from build123d import *

# Parameters (mm, degrees)
F1_DEPTH = 5.08
F2_SIZE  = 5.07999


# Not quite as in the source:
# - a fillet or chamfer is up to 0.001 mm smaller than in the source, because OpenCascade refuses the exact size


with BuildPart() as f1:
    # F0 (on Top) → F1 (new body)
    with BuildSketch(Plane.XY):
        with BuildLine():
            ThreePointArc((-6.4398498965, 10.9461560975), (-3.3372007403, 12.2536970429), (0, 12.7))
            Line((0, 12.7), (0, 38.1))
            Line((0, 38.1), (-11.0489271221, 18.7804503105))
            Line((-11.0489271221, 18.7804503105), (-6.4398498965, 10.9461560975))
        make_face()
        with BuildLine():
            ThreePointArc((0, 12.7), (3.261881723, 12.2739613665), (6.304915, 11.0244295473))
            Line((6.304915, 11.0244295473), (10.9721234563, 19.185255))
            Line((10.9721234563, 19.185255), (0, 38.1))
            Line((0, 38.1), (0, 12.7))
        make_face()
        with BuildLine():
            ThreePointArc((-2.7338674235, 4.6469001683), (-1.4167200379, 5.2019819875), (0, 5.3914480674))
            Line((0, 5.3914480674), (0, 12.7))
            ThreePointArc((0, 12.7), (-3.3372007403, 12.2536970429), (-6.4398498965, 10.9461560975))
            Line((-6.4398498965, 10.9461560975), (-2.7338674235, 4.6469001683))
        make_face()
        with BuildLine():
            ThreePointArc((0, 5.3914480674), (1.3847453474, 5.2105846684), (2.6765843931, 4.6801290848))
            Line((2.6765843931, 4.6801290848), (6.304915, 11.0244295473))
            ThreePointArc((6.304915, 11.0244295473), (3.261881723, 12.2739613665), (0, 12.7))
            Line((0, 12.7), (0, 5.3914480674))
        make_face()
        with BuildLine():
            ThreePointArc((-5.3914480674, 0), (-4.6801290848, 2.6765843931), (-2.7338674235, 4.6469001683))
            Line((-2.7338674235, 4.6469001683), (-6.4398498965, 10.9461560975))
            ThreePointArc((-6.4398498965, 10.9461560975), (-11.0244295473, 6.304915), (-12.7, 0))
            Line((-12.7, 0), (-5.3914480674, 0))
        make_face()
        with BuildLine():
            ThreePointArc((2.6765843931, 4.6801290848), (4.6636025783, 2.7052769276), (5.3914480674, 0))
            Line((5.3914480674, 0), (12.7, 0))
            ThreePointArc((12.7, 0), (10.9855, 6.3725026285), (6.304915, 11.0244295473))
            Line((6.304915, 11.0244295473), (2.6765843931, 4.6801290848))
        make_face()
        with BuildLine():
            Line((-10.9461560975, -6.4398498965), (-4.6469001683, -2.7338674235))
            ThreePointArc((-4.6469001683, -2.7338674235), (-5.2019819875, -1.4167200379), (-5.3914480674, 0))
            Line((-5.3914480674, 0), (-12.7, 0))
            ThreePointArc((-12.7, 0), (-12.2536970429, -3.3372007403), (-10.9461560975, -6.4398498965))
        make_face()
        with BuildLine():
            Line((12.7, 0), (5.3914480674, 0))
            ThreePointArc((5.3914480674, 0), (5.2105846684, -1.3847453474), (4.6801290848, -2.6765843931))
            Line((4.6801290848, -2.6765843931), (11.0244295473, -6.304915))
            ThreePointArc((11.0244295473, -6.304915), (12.2739613665, -3.261881723), (12.7, 0))
        make_face()
        with BuildLine():
            Line((11.0244295473, -6.304915), (4.6801290848, -2.6765843931))
            ThreePointArc((4.6801290848, -2.6765843931), (3.835671013, -3.7888441699), (2.7338674235, -4.6469001683))
            Line((2.7338674235, -4.6469001683), (6.4398498965, -10.9461560975))
            ThreePointArc((6.4398498965, -10.9461560975), (9.0352390037, -8.9249345178), (11.0244295473, -6.304915))
        make_face()
        with BuildLine():
            Line((6.4398498965, -10.9461560975), (2.7338674235, -4.6469001683))
            ThreePointArc((2.7338674235, -4.6469001683), (0.0331115783, -5.3913463891), (-2.6765843931, -4.6801290848))
            Line((-2.6765843931, -4.6801290848), (-6.304915, -11.0244295473))
            ThreePointArc((-6.304915, -11.0244295473), (0.07799705, -12.6997604883), (6.4398498965, -10.9461560975))
        make_face()
        with BuildLine():
            ThreePointArc((-2.6765843931, -4.6801290848), (-3.7888441699, -3.835671013), (-4.6469001683, -2.7338674235))
            Line((-4.6469001683, -2.7338674235), (-10.9461560975, -6.4398498965))
            ThreePointArc((-10.9461560975, -6.4398498965), (-8.9249345178, -9.0352390037), (-6.304915, -11.0244295473))
            Line((-6.304915, -11.0244295473), (-2.6765843931, -4.6801290848))
        make_face()
        with BuildLine():
            Line((-32.8384682925, -19.3195496895), (-10.9461560975, -6.4398498965))
            ThreePointArc((-10.9461560975, -6.4398498965), (-12.2536970429, -3.3372007403), (-12.7, 0))
            Line((-12.7, 0), (-21.7895411704, 0))
            Line((-21.7895411704, 0), (-32.8384682925, -19.3195496895))
        make_face()
        with BuildLine():
            ThreePointArc((-6.304915, -11.0244295473), (-8.9249345178, -9.0352390037), (-10.9461560975, -6.4398498965))
            Line((-10.9461560975, -6.4398498965), (-32.8384682925, -19.3195496895))
            Line((-32.8384682925, -19.3195496895), (-10.9721234563, -19.185255))
            Line((-10.9721234563, -19.185255), (-6.304915, -11.0244295473))
        make_face()
        with BuildLine():
            Line((33.0732886418, -18.914745), (11.0244295473, -6.304915))
            ThreePointArc((11.0244295473, -6.304915), (9.0352390037, -8.9249345178), (6.4398498965, -10.9461560975))
            Line((6.4398498965, -10.9461560975), (11.2069438057, -19.0490396895))
            Line((11.2069438057, -19.0490396895), (33.0732886418, -18.914745))
        make_face()
        with BuildLine():
            Line((22.1011651855, 0), (12.7, 0))
            ThreePointArc((12.7, 0), (12.2739613665, -3.261881723), (11.0244295473, -6.304915))
            Line((11.0244295473, -6.304915), (33.0732886418, -18.914745))
            Line((33.0732886418, -18.914745), (22.1011651855, 0))
        make_face()
    extrude(amount=F1_DEPTH)

    # F2 (size 5.08 in the source; OpenCascade refuses exactly that, so slightly less here)
    f2_edges = [f1.edges().sort_by_distance(p)[0] for p in [
        (-5.524464, 28.440225, 5.08),
        (5.486062, 28.642628, 5.08),
        (-27.314005, -9.659775, 5.08),
        (-21.905296, -19.252402, 5.08),
        (22.140116, -18.981892, 5.08),
        (27.587227, -9.457373, 5.08),
    ]]
    chamfer(f2_edges, length=F2_SIZE)


solid = f1.part
For this review, take the finished solid that the model builds, in its own axes (mm). A direction names the side the tool comes from. Coordinates: 2 decimals unless noted, no trailing zeros. Order: outer loops, then holes, each group sorted by start corner. A loop starts at its lowest first (then second) coordinate and runs counter-clockwise, first axis right, second up. Notation, with made-up numbers: (23, -31.5) - (38, -31.5) arc R24 ccw to (38, -13.5) - close; hole circle Ø7 at (49.25, 61). An arc over 180 degrees is marked (long way). Answer as CSV lines item,"result". Start each with the question number.
1) To check wall thickness, follow line 1 along X through (y, z) = (-4, 2.25); line 2 along X through (y, z) = (-4.5, 1.6); line 3 along Z through (x, y) = (24, -8.5). State the ranges of each line that lie inside material, in increasing order. Write a range as [from, to].
2) Machinability: for faces 1 (the flat face through (-8.153, -14.255, 1.94)), 2 (the cylindrical face through (-10.98, 6.38, 2.5)), 3 (the flat face through (8.087, 14.141, 1.94)), 4 (the flat face through (16, 0, 2)), which of the approach directions +Z, -Z, +X, -X, +Y, -Y give a long, thin tool a straight path to every point of the face, cutting with its end or side? Answer none if there is none.
3) Draft analysis for pull direction Y (two halves, no side actions). For faces 5 (the cylindrical face through (11.032, 6.291, 2.504)), 6 (the flat face through (8.26, -14.04, 1.94)), 7 (the flat face through (-16, 0, 2)), state which applies: +Y half, -Y half, draft (parallel to the pull), parting line (faces both ways), or undercut.
4) Insertion check: P1, Ø2, axis at y = 29, z = 2, coming from the +X side; P2, Ø2, axis at y = 28, z = 3, coming from the -X side; P3, Ø2.5, axis at x = -15.5, z = 3.5, coming from the +Y side; P4, Ø8, axis at x = 7, y = 18, coming from the +Z side. Each pin has a flat end and moves straight along its axis. Give the tip position at first contact, or say it passes through.
5) Add section C-C (y = 16.5). State the section outline as (x, z) points, then the cut area to 3 significant figures.
6) Add section B-B (z = 2.15). State the section outline as (x, y) points.
Result:
1,line 1,"[-21.49, -3.61], [3.61, 21.82]"
1,line 2,"[-22.52, -2.97], [2.97, 22.86]"
1,line 3,"[0, 2.62]"
2,face 1,"+Z, -Z, -Y"
2,face 2,"+Z, -Z, -X"
2,face 3,"+Z, -Z, +X"
2,face 4,"+Z, -Z, +X, +Y"
3,face 5,"undercut"
3,face 6,"-Y half"
3,face 7,"+Y half"
4,P1,"x = 4.26"
4,P2,"x = -3.61"
4,P3,"y = 0"
4,P4,"z = 5.08"
5,outline,"(-9.71, 0) - (9.44, 0) - (9.44, 2.68) - (6.66, 5.08) - (-6.5, 5.08) - (-9.71, 2.3) - close"
5,area,"89.4 mm^2"
6,outline,"(-29.12, -17.15) - (-9.74, -17.03) - (-6.3, -11.02) arc R12.7 ccw to (6.44, -10.95) - (9.95, -16.91) - (29.35, -16.79) - (19.62, 0) - (12.7, 0) arc R12.7 ccw to (6.3, 11.02) - (9.74, 17.03) - (0.01, 33.79) - (-9.79, 16.65) - (-6.44, 10.95) arc R12.7 ccw to (-12.7, 0) - (-19.31, 0) - close; hole circle Ø10.78 at (0, 0)"
